from build123d import *

# Parameters (mm, degrees)
SKETCH_W     = 5
SKETCH_H     = 1.2
PAD_DEPTH    = 9.8
POCKET_DEPTH = 9.801


with BuildPart() as part:
    # Sketch → Pad (new body)
    with BuildSketch(Plane.XY):
        Polygon((-26.871767, -5.673633), (-56.871767, -5.673633), (-56.871767, -10.473633), (-21.871767, -10.473633), (39.628233, -5.673633), (39.628233, 19.326367), (29.628233, 19.326367), (29.628233, 14.326367), (34.628233, 14.326367), (34.628233, -0.673633), (-26.871767, -0.673633), align=None)
        with Locations((-49.371767, -8.073633)):
            Rectangle(SKETCH_W, SKETCH_H, mode=Mode.SUBTRACT)
    extrude(amount=PAD_DEPTH)

    # Sketch001 → Pocket (cut, through all)
    with BuildSketch(Plane.XY.offset(9.8)):
        Polygon((-21.871767, -4.405271), (-21.871767, -5.465759), (-2.982301, -4.405271), align=None)
    extrude(amount=-POCKET_DEPTH, mode=Mode.SUBTRACT)


solid = part.part
Design review of the part built by this model. Coordinates are the model's own, in mm. A direction names the side the tool comes from. Round coordinates to 2 decimals unless told otherwise and drop trailing zeros. Write each loop counter-clockwise with the first axis right and the second up, starting at its lowest first coordinate (ties: lowest second). Pieces come first, ordered by that corner, then holes. Notation, with made-up numbers: M 58.25,39.25 L 84.25,39.25 A23 ccw 84.25,64.25 Z; hole C 29,13 d4. An arc over 180 degrees is marked long. One line per item, written item: value. Start each with the question number.
1. Take a section at D-D on x = -28. State the section outline as (y, z) points.
2. For faces 1 (the face through (-26.872, -3, 5)), 2 (the face through (-40, -10.474, 5)), 3 (the face through (-2, -1, 0)), 4 (the face through (34.628, 7, 5)), 5 (the face through (-49, -7.474, 5)), list the 3-axis set-ups (+Z, -Z, +X, -X, +Y, -Y) from which the entire face can be reached by the end or side of a thin tool; tool diameter is ignored.
3. To check wall thickness, follow probe 1 along Y at (x, z) = (-47.5, 3.5); probe 2 along X at (y, z) = (13.5, 1.5); probe 3 along X at (y, z) = (18, 7.5). State the ranges of each line that lie inside material, in increasing order. Write a range as from..to.
4. Take a section at C-C on y = 8.5. State the section outline as (x, z) points.
5. Clearance check with flat-ended pins moving along their axes: P1, Ø4, axis at x = -5.5, y = 1.5, coming from the +Z side; P2, Ø5, axis at y = 8, z = 5, coming from the -X side; P3, Ø5, axis at x = -46, z = 6.5, coming from the +Y side; P4, Ø4, axis at x = 20, z = 6, coming from the +Y side. State where each tip first meets the part, or that it passes through.
6. Draft analysis for pull direction Y (two halves, no side actions). For faces 6 (the face through (-42, -5.674, 5)), 7 (the face through (39.628, 7, 5)), 8 (the face through (-12.559, -4.943, 4.969)), state which applies: pulls with the +Y half, pulls with the -Y half, needs draft (parallel to the pull), parting line crosses it, or undercut.
7. Take a section at A-A on z = 3.25. State the section outline as (x, y) points.
8. Take a section at B-B on x = 33.5. State the section outline as (y, z) points, then the cut area to 3 significant figures.
Computed:
1. outline: M -10.47,0 L -5.67,0 L -5.67,9.8 L -10.47,9.8 Z
2. face 1: +Z, -Z, -X, +Y
2. face 2: +Z, -Z, +X, -X, -Y
2. face 3: -Z, +X, -X, +Y, -Y
2. face 4: +Z, -Z, -X
2. face 5: +Z, -Z
3. probe 1: y = -10.47..-8.67, -7.47..-5.67
3. probe 2: x = 34.63..39.63
3. probe 3: x = 29.63..39.63
4. outline: M 34.63,0 L 39.63,0 L 39.63,9.8 L 34.63,9.8 Z
5. P1: passes through
5. P2: stops at x = 34.63
5. P3: stops at y = -5.67
5. P4: stops at y = -0.67
6. face 6: pulls with the +Y half
6. face 7: needs draft
6. face 8: undercut
7. outline: M -56.87,-10.47 L -21.87,-10.47 L 39.63,-5.67 L 39.63,19.33 L 29.63,19.33 L 29.63,14.33 L 34.63,14.33 L 34.63,-0.67 L -26.87,-0.67 L -26.87,-5.67 L -56.87,-5.67 Z; hole M -51.87,-8.67 L -46.87,-8.67 L -46.87,-7.47 L -51.87,-7.47 Z; hole M -21.87,-5.47 L -2.98,-4.41 L -21.87,-4.41 Z
8. outline: M -6.15,0 L -0.67,0 L -0.67,9.8 L -6.15,9.8 Z; M 14.33,0 L 19.33,0 L 19.33,9.8 L 14.33,9.8 Z
8. area: 103 mm²
